Autodesk Inventor part; units mm, degrees
ref_plane "YZ Plane" through (0, 0, 0) normal (1, 0, 0) x (0, 1, 0)
ref_plane "XZ Plane" through (0, 0, 0) normal (0, 1, 0) x (-1, 0, 0)
ref_plane "XY Plane" through (0, 0, 0) normal (0, 0, 1) x (1, 0, 0)
sketch "Náčrt1" plane through (0, 0, 0) normal (0, 1, 0) x (-1, 0, 0)
  line L0 (0, -63) -> (0, 63)
  line L1 (-63, 0) -> (63, 0)
  line L2 (45, 45) -> (-45, 45)
  line L3 (-45, 45) -> (-45, -45)
  line L4 (-45, -45) -> (45, -45)
  line L5 (45, -45) -> (45, 45)
  point P0 (0, 0)
  dimension "d0" = 90
  dimension "d1" = 90
extrude "Vysunutí1" add sketch "Náčrt1" along normal blind 3
sketch "Náčrt2" plane through (0, 3, 0) normal (0, 1, 0) x (1, 0, 0)
  line L0 (0, 63) -> (0, -63)
  line L1 (63, 0) -> (-63, 0)
  line L2 (-41.5, -42) -> (-12.5, -42)
  line L3 (-12.5, -42) -> (-12.5, 42)
  line L4 (-12.5, 42) -> (-41.5, 42)
  line L5 (-41.5, 42) -> (-41.5, -42)
  line L6 (-45, 45) -> (-45, -45)
  point P0 (0, 0)
  dimension "d4" = 3.5
  dimension "d5" = 29
  dimension "d6" = 84
extrude "Vysunutí2" add sketch "Náčrt2" along normal blind 3
sketch "Náčrt3" plane through (0, 3, 0) normal (0, 1, 0) x (1, 0, 0)
  line L0 (-12.5, -42) -> (-12.5, 42)
  line L1 (0, 63) -> (0, -63)
  line L2 (63, 0) -> (-63, 0)
  line L3 (-6.5, -42) -> (42.5, -42)
  line L4 (42.5, -42) -> (42.5, 42)
  line L5 (42.5, 42) -> (-6.5, 42)
  line L6 (-6.5, 42) -> (-6.5, -42)
  point P0 (0, 0)
  point P1 (18, -42)
  dimension "d9" = 6
  dimension "d10" = 49
  dimension "d11" = 84
extrude "Vysunutí3" add sketch "Náčrt3" along normal blind 3
sketch "Náčrt6" plane through (0, 0, 0) normal (0, -1, 0) x (1, 0, 0)
  line L0 (0, 63) -> (0, -63)
  line L1 (-63, 0) -> (63, 0)
  line L2 (-10, 0) -> (10, 0) construction
  line L3 (-6.5, -42) -> (-6.5, 42)
  line L4 (-10, -2.5) -> (10, -2.5)
  line L5 (10, 2.5) -> (-10, 2.5)
  arc A0 (-10, 2.5) -> (-10, -2.5) centre (-10, 0) ccw
  arc A1 (10, -2.5) -> (10, 2.5) centre (10, 0) ccw
  point P0 (0, 0)
  point P1 (0, 0)
  dimension "d14" = 20
  dimension "d15" = 5
extrude "Vysunutí4" add sketch "Náčrt6" along normal blind 5
properties part number "víčko"
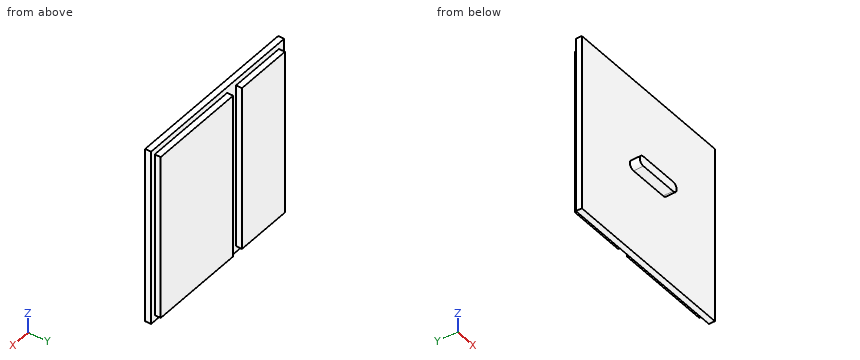
Design review of the part built by this model. Coordinates are the model's own, in mm. Give positions to 0.01 mm unless a question says otherwise; leave off trailing zeros. Order: outer loops, then holes, each group sorted by start corner. A loop starts at its lowest first (then second) coordinate and runs counter-clockwise, first axis right, second up. Notation, with made-up numbers: (-10.5, 20.25) - (46.5, 20.25) arc R10 cw to (46.5, 27.25) - close; hole circle Ø10 at (83, 79.25). An arc over 180 degrees is marked (long way). Use a Markdown table: item, result. Add a question column.
(1) Clearance check with flat-ended pins moving along their axes: P1, Ø2.5, axis at x = -2, y = -2.5, coming from the -Z side; P2, Ø3, axis at x = -31.5, z = 25, coming from the -Y side; P3, Ø3.5, axis at y = 5, z = 17, coming from the +X side. State where each tip first meets the part, or that it passes through.
(2) Add section C-C on x = -24. Give the boundary of the cut face in (y, z).
(3) Add section A-A on y = 4.75. Give the boundary of the cut face in (x, z).
(4) Add section B-B on z = 0. Give the boundary of the cut face in (x, y), then the cut area to 3 significant figures.
(5) Wall thickness on probe 1 along X at (y, z) = (3.5, 31.5); probe 2 along Y at (x, z) = (-31, 10); probe 3 along Z at (x, y) = (-7, -2.25): over which ranges is each line inside the solid? List them lowest first. Write a range as [from, to].
(6) Add section D-D on z = 31. Give the boundary of the cut face in (x, y).
Report:
| question | item | result |
|---|---|---|
| 1 | P1 | stops at z = -2.5 |
| 1 | P2 | stops at y = 0 |
| 1 | P3 | stops at x = 42.5 |
| 2 | outline | (0, -45) - (3, -45) - (3, -42) - (6, -42) - (6, 42) - (3, 42) - (3, 45) - (0, 45) - close |
| 3 | outline | (-41.5, -42) - (-12.5, -42) - (-12.5, 42) - (-41.5, 42) - close; (-6.5, -42) - (42.5, -42) - (42.5, 42) - (-6.5, 42) - close |
| 4 | outline | (-45, 0) - (-12.5, 0) - (-12.5, -5) - (12.5, -5) - (12.5, 0) - (45, 0) - (45, 3) - (42.5, 3) - (42.5, 6) - (-6.5, 6) - (-6.5, 3) - (-12.5, 3) - (-12.5, 6) - (-41.5, 6) - (-41.5, 3) - (-45, 3) - close |
| 4 | area | 629 mm² |
| 5 | probe 1 | x = [-41.5, -12.5], [-6.5, 42.5] |
| 5 | probe 2 | y = [0, 6] |
| 5 | probe 3 | z = [-2.5, 2.5] |
| 6 | outline | (-45, 0) - (45, 0) - (45, 3) - (42.5, 3) - (42.5, 6) - (-6.5, 6) - (-6.5, 3) - (-12.5, 3) - (-12.5, 6) - (-41.5, 6) - (-41.5, 3) - (-45, 3) - close |
